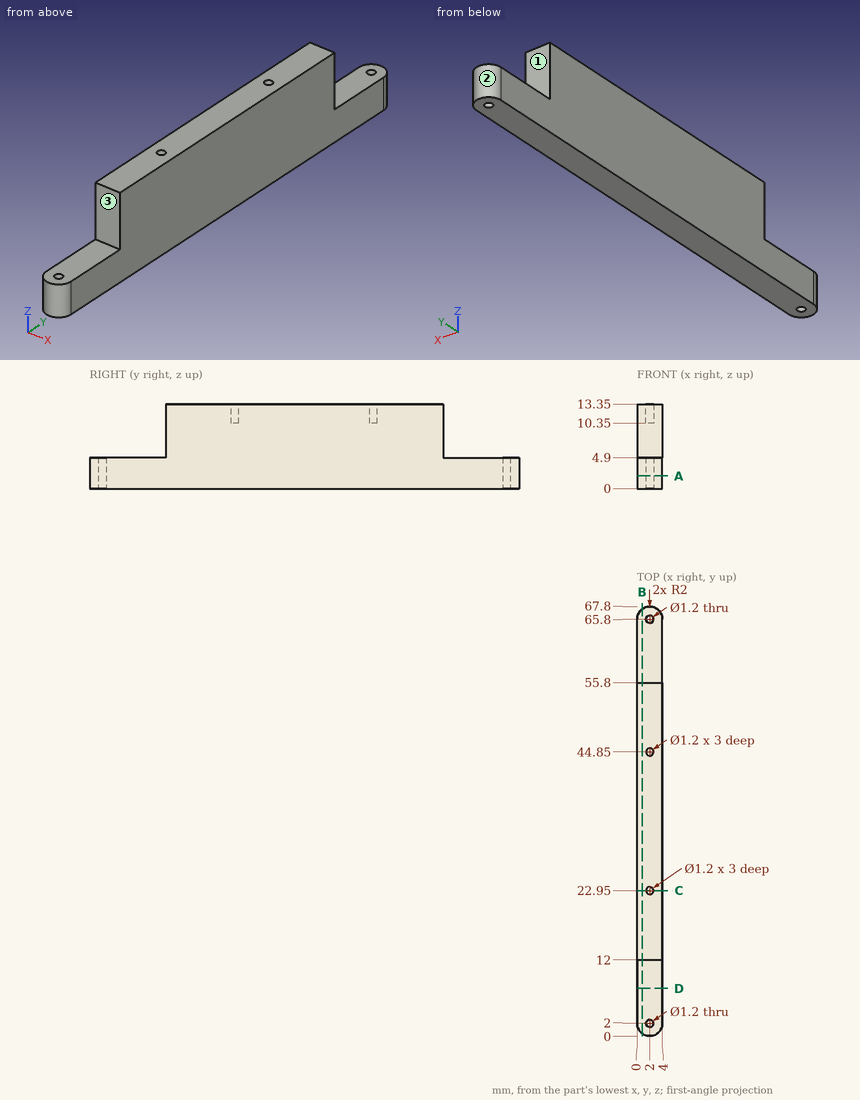
Geometry check sheet. Reference: drawing and pictorial views, mm from the part's lowest x, y, z. A direction names the side the tool comes from. Give positions to 0.01 mm unless a question says otherwise; leave off trailing zeros. Write each loop counter-clockwise with the first axis right and the second up, starting at its lowest first coordinate (ties: lowest second). Pieces come first, ordered by that corner, then holes. Notation, with made-up numbers: (53, -38.75) -> (79, -38.75) arc R15 ccw to (79, -13.75) -> close; hole circle Ø1 at (12.5, -5.75). An arc over 180 degrees is marked (long way). One line per question, with ' | ' between items.
Item 1: Access from +Z, -Z, +X, -X, +Y, -Y to the whole of each face (thin tool, end or side, straight path). Record for the marked faces 1, 2 and 3.
Determined:
face 1: +Z, +X, -X, +Y | face 2: +Z, -Z, +Y | face 3: +Z, +X, -X, -Y
Item 2: Sectioned sample at C-C, the plane y = 22.95. Record the boundary of the cut face in (x, z), plus the area to 3 significant figures.
Determined:
outline: (0, 0) -> (4, 0) -> (4, 13.35) -> (2.6, 13.35) -> (2.6, 10.35) -> (1.4, 10.35) -> (1.4, 13.35) -> (0, 13.35) -> close | area: 49.8 mm^2
Item 3: Scan lines: line 1 along Y through (x, z) = (2, 12); line 2 along Y through (x, z) = (2, 1.35); line 3 along Y through (x, z) = (3.15, 12.25). Record each from-to range of solid material in increasing order.
Determined:
line 1: 12 to 22.35, 23.55 to 44.25, 45.45 to 55.8 | line 2: 0 to 1.4, 2.6 to 65.2, 66.4 to 67.8 | line 3: 12 to 55.8
Item 4: Sectioned sample at A-A, the plane z = 2. Record the boundary of the cut face in (x, y).
Determined:
outline: (0, 2) arc R2 ccw to (4, 2) -> (4, 65.8) arc R2 ccw to (0, 65.8) -> close; hole circle Ø1.2 at (2, 2); hole circle Ø1.2 at (2, 65.8)
Item 5: Depth check by flat-ended pin: pin 1 (2 mm diameter, centred on x = 1, z = 11, fed in from +Y); pin 2 (1.2 mm diameter, centred on x = 3, y = 6.5, fed in from +Z). Enter the tip coordinate at first touch or a pass-through.
Determined:
pin 1: y = 55.8 | pin 2: z = 4.9
Item 6: Sectioned sample at B-B, the plane x = 0.8. Record the boundary of the cut face in (y, z), plus the area to 3 significant figures.
Determined:
outline: (0.4, 0) -> (67.4, 0) -> (67.4, 4.9) -> (55.8, 4.9) -> (55.8, 13.35) -> (12, 13.35) -> (12, 4.9) -> (0.4, 4.9) -> close | area: 698 mm^2
Item 7: Sectioned sample at D-D, the plane y = 7.5. Record the boundary of the cut face in (x, z).
Determined:
outline: (0, 0) -> (4, 0) -> (4, 4.9) -> (0, 4.9) -> close
